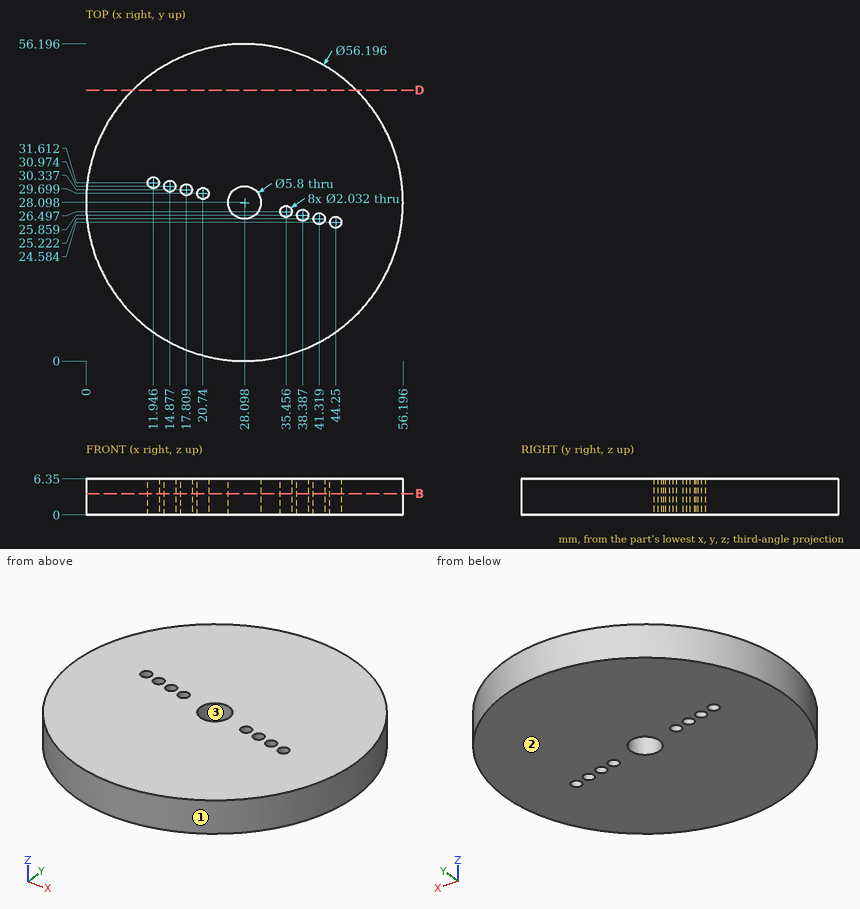
Geometry: see drawing. Coordinates: mm, zero at the bounding-box minimum. Give positions to 0.01 mm unless a question says otherwise; leave off trailing zeros. Loops run counter-clockwise (first coordinate to the right, second up) from the corner with the lowest first, then second, coordinate; pieces in that order, holes last. Notation, with made-up numbers: M -29.5,15.25 L 18.5,15.25 A34 cw 18.5,51.25 Z; hole C 74.25,22 d9. An arc over 180 degrees is marked long. Answer as CSV lines item,"result". Start each with the question number.
1. Section D-D on y = 48. Return loops of the section in (x, z), plus the area to 3 significant figures.
2. Pin query (flat end, axial travel): P1, Ø2, axis at x = 26.5, z = 4, coming from the -Y side; P2, Ø1.5, axis at x = 39, z = 0.5, coming from the -Y side. Return the tip coordinate at first contact, or that it passes through.
3. Pull-direction query (Y, two-part tool) for the marked faces 1, 2 and 3; classes: released by +Y, released by -Y, zero draft, split by the parting line, or undercut.
4. Section B-B on z = 3.75. State how many separate pieces and enclosed holes the cut face has, plus the area to 3 significant figures.
5. Line query: L1, parallel to X at y = 25, z = 1 (1 decimal); L2, parallel to Y at x = 30, z = 0.75 (1 decimal); L3, parallel to Y at x = 44.5, z = 2.5 (1 decimal). Output: solid intervals per line, ascending.
Computed values:
1,outline,"M 8.26,0 L 47.93,0 L 47.93,6.35 L 8.26,6.35 Z"
1,area,"252 mm²"
2,P1,"stops at y = 0.01"
2,P2,"stops at y = 1.9"
3,face 1,"split by the parting line"
3,face 2,"zero draft"
3,face 3,"undercut"
4,separate pieces,"1"
4,enclosed holes,"9"
4,area,"2,430 mm²"
5,L1,"x = 0.2 to 37.8, 38.9 to 40.3, 42.3 to 43.3, 45.2 to 56"
5,L2,"y = 0.1 to 25.9, 30.3 to 56.1"
5,L3,"y = 5.3 to 23.6, 25.6 to 50.9"
